from build123d import *

# Parameters (mm, degrees)
SKETCH1_R           = 37.85
BOSS_EXTRUDE1_DEPTH = 19.4
SKETCH4_R           = 1.5
CUT_EXTRUDE1_DEPTH  = 1


with BuildPart() as part:
    # Sketch1 → Boss-Extrude1 (new body)
    with BuildSketch(Plane(origin=(0, 0, 0), x_dir=(1, 0, 0), z_dir=(0, 1, 0))):
        with Locations(Location((0, 0, 0), (0, 0, 270))):
            Circle(SKETCH1_R)
    extrude(amount=BOSS_EXTRUDE1_DEPTH)

    # Sketch3 → Revolve1 (revolve)
    with BuildSketch(Plane(origin=(0, 0, 0), x_dir=(0, 0, -1), z_dir=(1, 0, 0))):
        with BuildLine():
            Line((37.85, 19.4), (37.85, 30.8))
            Line((37.85, 30.8), (37.85, 31.91000006))
            ThreePointArc((37.85, 31.91000006), (35.246179285, 38.196179345), (28.96, 40.80000006))
            Line((28.96, 40.80000006), (0, 40.80000006))
            Line((0, 40.80000006), (0, 19.4))
            Line((0, 19.4), (37.85, 19.4))
        make_face()
    revolve(axis=Axis((0, 19.4, 0), (0, 1, 0)))

    # Sketch4 → Cut-Extrude1 (cut)
    with BuildSketch(Plane.XZ):
        with Locations(Location((20.859650045, 20.859650045, 0), (0, 0, 270))):
            Circle(SKETCH4_R)
        with Locations(Location((-20.859650045, 20.859650045, 0), (0, 0, 270))):
            Circle(SKETCH4_R)
        with Locations(Location((-20.859650045, -20.859650045, 0), (0, 0, 270))):
            Circle(SKETCH4_R)
        with Locations(Location((20.859650045, -20.859650045, 0), (0, 0, 270))):
            Circle(SKETCH4_R)
    extrude(amount=-CUT_EXTRUDE1_DEPTH, mode=Mode.SUBTRACT)


solid = part.part
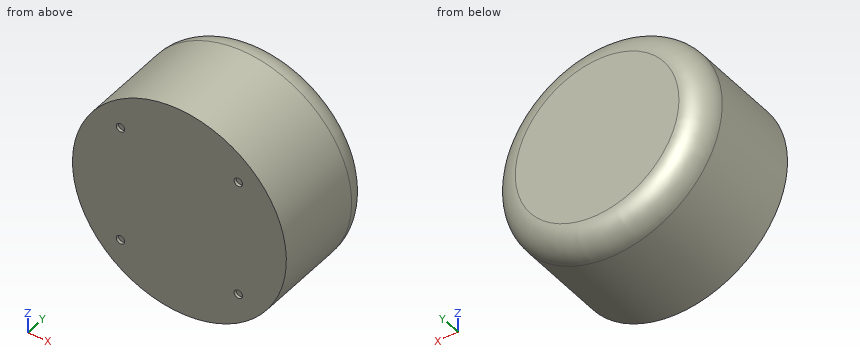
Work out the finished part from the listing and answer in its coordinate system (mm). Round coordinates to 2 decimals unless told otherwise and drop trailing zeros. Write each loop counter-clockwise with the first axis right and the second up, starting at its lowest first coordinate (ties: lowest second). Pieces come first, ordered by that corner, then holes.
1) Given pin 1 Ø6 at (x, y) = (-16, 24) entering from -Z; pin 2 Ø1.8 at (x, z) = (20.86, -20.86) entering from -Y; pin 3 Ø8 at (y, z) = (9.5, 10.5) entering from +X, each flat-ended and moving along its own axis, determine where each tip first touches the part or whether it passes through.
2) A cutting plane is placed at A-A (y = 14.5). Give the vertices of the cut face in (x, z), plus the area to 3 significant figures.
3) Straight lines are drawn through the part: line 1 (X direction, y = 36, z = -0.5); line 2 (Z direction, x = -25.5, y = 7.5); line 3 (Z direction, x = -13, y = 4). For each, find the intervals that lie inside material, in ascending order.
Completed:
1. pin 1: stops at z = -35.55
1. pin 2: stops at y = 1
1. pin 3: stops at x = 37.29
2. outline: circle Ø75.7 at (0, 0)
2. area: 4,500 mm2
3. line 1: x = -36.85 to 36.85
3. line 2: z = -27.97 to 27.97
3. line 3: z = -35.55 to 35.55
